Work out the finished part from the listing and answer in its coordinate system (mm). A direction names the side the tool comes from. Coordinates: 2 decimals unless noted, no trailing zeros. Order: outer loops, then holes, each group sorted by start corner. A loop starts at its lowest first (then second) coordinate and runs counter-clockwise, first axis right, second up.
1. A tool of negligible diameter and unlimited length cuts with its end or side. For faces 4 (the cylindrical face through (-6.2, 31.63, -1.1)), 5 (the flat face through (-12.573, 27, 0)), from which of +Z, -Z, +X, -X, +Y, -Y can it reach the whole face along a straight path? Write none if from no direction.
2. The part is cut by section C-C, the plane z = 4.5. Give the vertices of the cut face in (x, y), then the cut area to 3 significant figures.
3. The part is cut by section B-B, the plane x = 7.5. Give the vertices of the cut face in (y, z).
4. Determine the mould class of faces 1 (the flat face through (8, 0, 0)), 2 (the flat face through (12.7, 9, 0)), 3 (the cylindrical face through (19.045, 17.531, -0.419)) for opening direction Z: +Z half, -Z half, draft (parallel to the pull), parting line (faces both ways), or undercut.
5. The part is cut by section A-A, the plane y = 26.67. Give the vertices of the cut face in (x, z).
6. Flat-ended cylindrical pins translate along their axes: pin 1 Ø12 at (y, z) = (8.89, 0) entering from -X; pin 2 Ø2 at (x, y) = (-6.5, 27) entering from -Z; pin 3 Ø4 at (y, z) = (29.5, -6.5) entering from +X. Find the tip coordinate at first contact, or state that the pin passes through.
7. The part is cut by section D-D, the plane y = 8.89. Give the vertices of the cut face in (x, z).
8. Find the intervals of material crossed by probe 1 along Y at (x, z) = (7.75, 0); probe 2 along X at (y, z) = (19, 16.5); probe 3 along Z at (x, y) = (-11, 29.5), in increasing order.
Autodesk Inventor part; units mm, degrees
ref_plane "YZ Plane" through (0, 0, 0) normal (1, 0, 0) x (0, 1, 0)
ref_plane "XZ Plane" through (0, 0, 0) normal (0, 1, 0) x (-1, 0, 0)
ref_plane "XY Plane" through (0, 0, 0) normal (0, 0, 1) x (1, 0, 0)
sketch "Sketch1" plane through (0, 0, 0) normal (0, 1, 0) x (-1, 0, 0)
  arc A0 (0, 19.05) -> (0, -19.05) centre (0, 0) ccw
  line L0 (0, 19.05) -> (0, -19.05)
  dimension "d0" = 38.1
extrude "Extrusion1" add sketch "Sketch1" along normal blind 35.56
sketch "Sketch2" plane through (0, 0, -19.05) normal (-1, 0, 0) x (0, 0, 1)
  line L0 (0, 35.56) -> (38.1, 35.56)
  line L1 (0, 0) -> (0, 35.56)
  circle A0 centre (19.05, 26.67) radius 5.08
  circle A1 centre (19.05, 8.89) radius 5.207
  point P0 (19.05, 0)
  dimension "d6" = 10.414
extrude "Extrusion2" cut sketch "Sketch2" against normal blind 12.7 contours A1
extrude "Extrusion3" add sketch "Sketch2" along normal blind 12.573 contours A0
properties part number "Piston Mold"
Geometry says:
1. face 4: -X
1. face 5: +Z, -Z, -X, +Y, -Y
2. outline: (-12.57, 24.31) - (0, 24.31) - (0, 11.51) - (12.7, 11.51) - (12.7, 6.27) - (0, 6.27) - (0, 0) - (18.51, 0) - (18.51, 35.56) - (0, 35.56) - (0, 29.03) - (-12.57, 29.03) - close
2. area: 651 mm2
3. outline: (0, -17.51) - (35.56, -17.51) - (35.56, 17.51) - (0, 17.51) - close; hole circle Ø10.41 at (8.89, 0)
4. face 1: draft
4. face 2: undercut
4. face 3: parting line
5. outline: (-12.57, -5.08) - (0, -5.08) - (0, -19.05) arc R19.05 ccw to (0, 19.05) - (0, 5.08) - (-12.57, 5.08) - close
6. pin 1: stops at x = 0
6. pin 2: stops at z = -5.08
6. pin 3: stops at x = 18.51
7. outline: (0, -19.05) arc R19.05 ccw to (0, 19.05) - (0, 5.21) - (12.7, 5.21) - (12.7, -5.21) - (0, -5.21) - close
8. probe 1: y = 0 to 3.68, 14.1 to 35.56
8. probe 2: x = 0 to 9.52
8. probe 3: z = -4.22 to 4.22
